```python
from build123d import *

# Parameters (mm, degrees)
BOSS_EXTRUDE1_DEPTH = 4
SKETCH3_R           = 3.1
CUT_EXTRUDE1_DEPTH  = 1
SKETCH4_R           = 2.4
CUT_EXTRUDE2_DEPTH  = 22.365860619
CUT_EXTRUDE4_START  = -1
SKETCH7_R           = 3.1
CUT_EXTRUDE4_DEPTH  = 1
LPATTERN3_COUNT     = 3
LPATTERN3_PITCH     = 8
CUT_EXTRUDE5_DEPTH  = 22.365860619
LPATTERN4_COUNT     = 2
LPATTERN4_PITCH     = 8


with BuildPart() as part:
    # Sketch2 → Boss-Extrude1 (new, symmetric)
    with BuildSketch(Plane(origin=(0, 0, 0), x_dir=(1, 0, 0), z_dir=(0, 1, 0))):
        with BuildLine():
            Line((0, 3.5), (16, 3.5))
            ThreePointArc((16, 3.5), (19.5, 0), (16, -3.5))
            Line((16, -3.5), (0, -3.5))
            ThreePointArc((0, -3.5), (-3.5, 0), (0, 3.5))
        make_face()
    extrude(amount=BOSS_EXTRUDE1_DEPTH, both=True)

    # Sketch3 → Cut-Extrude1 (cut)
    with BuildSketch(Plane(origin=(0, 4, 0), x_dir=(1, 0, 0), z_dir=(0, 1, 0))):
        with Locations(Location((0, 0, 0), (0, 0, 270))):
            Circle(SKETCH3_R)
    cut_extrude1 = extrude(amount=-CUT_EXTRUDE1_DEPTH, mode=Mode.SUBTRACT)

    # Sketch4 → Cut-Extrude2 (cut, through all)
    with BuildSketch(Plane(origin=(0, 4, 0), x_dir=(1, 0, 0), z_dir=(0, 1, 0))):
        with Locations(Location((0, 0, 0), (0, 0, 270))):
            Circle(SKETCH4_R)
    cut_extrude2 = extrude(amount=-CUT_EXTRUDE2_DEPTH, mode=Mode.SUBTRACT)

    # Sketch7 → Cut-Extrude4 (cut)
    with BuildSketch(Plane(origin=(0, -4, 0), x_dir=(-1, 0, 0), z_dir=(0, -1, 0)).offset(CUT_EXTRUDE4_START)):
        with Locations(Location((0, 0, 0), (0, 0, 270))):
            Circle(SKETCH7_R)
    cut_extrude4 = extrude(amount=CUT_EXTRUDE4_DEPTH, mode=Mode.SUBTRACT)

    # LPattern3: Cut-Extrude1, Cut-Extrude2, Cut-Extrude4 ×3
    with Locations(*[(i * LPATTERN3_PITCH, 0, 0) for i in range(1, LPATTERN3_COUNT)]):
        add(cut_extrude1, mode=Mode.SUBTRACT)
        add(cut_extrude2, mode=Mode.SUBTRACT)
        add(cut_extrude4, mode=Mode.SUBTRACT)

    # Sketch8 → Cut-Extrude5 (cut, through all)
    with BuildSketch(Plane(origin=(0, 4, 0), x_dir=(1, 0, 0), z_dir=(0, 1, 0))):
        with BuildLine():
            Line((2.814249456, 3.1), (5.185750544, 3.1))
            ThreePointArc((5.185750544, 3.1), (5.553697029, 2.856892908), (5.474391514, 2.423076923))
            ThreePointArc((5.474391514, 2.423076923), (4.5, 0), (5.474391514, -2.423076923))
            ThreePointArc((5.474391514, -2.423076923), (5.553697029, -2.856892908), (5.185750544, -3.1))
            Line((5.185750544, -3.1), (2.814249456, -3.1))
            ThreePointArc((2.814249456, -3.1), (2.446302971, -2.856892908), (2.525608486, -2.423076923))
            ThreePointArc((2.525608486, -2.423076923), (3.5, 0), (2.525608486, 2.423076923))
            ThreePointArc((2.525608486, 2.423076923), (2.446302971, 2.856892908), (2.814249456, 3.1))
        make_face()
    cut_extrude5 = extrude(amount=-CUT_EXTRUDE5_DEPTH, mode=Mode.SUBTRACT)

    # LPattern4: Cut-Extrude5 ×2
    with Locations(*[(i * LPATTERN4_PITCH, 0, 0) for i in range(1, LPATTERN4_COUNT)]):
        add(cut_extrude5, mode=Mode.SUBTRACT)


solid = part.part
```
Verification items for the finished model (mm, model axes). A direction names the side the tool comes from. Coordinates: 2 decimals unless noted, no trailing zeros. Loops run counter-clockwise (first coordinate to the right, second up) from the corner with the lowest first, then second, coordinate; pieces in that order, holes last. Notation, with made-up numbers: (76, -9) - (102, -9) arc R29 ccw to (102, 24) - close; hole circle Ø2 at (-8, 82.25). An arc over 180 degrees is marked (long way). Put each result on its own line as item: value.
Item 1: Gauge pin test, flat ends, axial feed: pin 1 Ø1.5 at (y, z) = (-3, 1) entering from +X; pin 2 Ø3 at (x, z) = (8.5, -1) entering from -Y. Record the tip position at first contact, or that the pin passes through.
Conclusion:
pin 1: stops at x = 19.49
pin 2: stops at y = -3
Item 2: Section check B-B (y = -0.5). Enter the section's corners in (x, z), then the cut area to 3 significant figures.
Conclusion:
outline: (0, -3.5) - (16, -3.5) arc R3.5 ccw to (16, 3.5) - (0, 3.5) arc R3.5 ccw to start; hole circle Ø4.8 at (0, 0); hole (2.53, -2.42) arc R0.4 ccw to (2.81, -3.1) - (5.19, -3.1) arc R0.4 ccw to (5.47, -2.42) arc R3.5 cw to (5.47, 2.42) arc R0.4 ccw to (5.19, 3.1) - (2.81, 3.1) arc R0.4 ccw to (2.53, 2.42) arc R3.5 cw to start; hole circle Ø4.8 at (8, 0); hole (10.53, -2.42) arc R0.4 ccw to (10.81, -3.1) - (13.19, -3.1) arc R0.4 ccw to (13.47, -2.42) arc R3.5 cw to (13.47, 2.42) arc R0.4 ccw to (13.19, 3.1) - (10.81, 3.1) arc R0.4 ccw to (10.53, 2.42) arc R3.5 cw to start; hole circle Ø4.8 at (16, 0)
area: 72.4 mm2
Item 3: Scan lines: line 1 along X through (y, z) = (-1, 0); line 2 along X through (y, z) = (-3.45, 0); line 3 along Z through (x, y) = (0, -3.5). Record each from-to range of solid material in increasing order.
Conclusion:
line 1: x = -3.5 to -2.4, 2.4 to 3.5, 4.5 to 5.6, 10.4 to 11.5, 12.5 to 13.6, 18.4 to 19.5
line 2: x = -3.5 to -3.1, 3.1 to 3.5, 4.5 to 4.9, 11.1 to 11.5, 12.5 to 12.9, 19.1 to 19.5
line 3: z = -3.5 to -3.1, 3.1 to 3.5
Item 4: Set-up check for faces 1 (the face through (6, 3, 2)), 2 (the face through (4.5, 0.1, 0)), 3 (the face through (18, -3, 2)), 4 (the face through (10, -4, -3)), 5 (the face through (10, 4, -3)): record each of +Z, -Z, +X, -X, +Y, -Y from which the full face is reachable in a straight line by a thin tool's end or side.
Conclusion:
face 1: +Y
face 2: +Y, -Y
face 3: -Y
face 4: +Z, -Z, +X, -X, -Y
face 5: +Z, -Z, +X, -X, +Y
Item 5: Section check C-C (z = 0). Give the number of separate pieces and of enclosed holes in the cut face, then the cut area to 3 significant figures.
Conclusion:
separate pieces: 6
enclosed holes: 0
area: 44.4 mm2
Item 6: Section check D-D (x = -1.75). Enter the section's corners in (y, z), then the cut area to 3 significant figures.
Conclusion:
outline: (-4, -3.03) - (4, -3.03) - (4, -2.56) - (3, -2.56) - (3, -1.64) - (-3, -1.64) - (-3, -2.56) - (-4, -2.56) - close; (-4, 2.56) - (-3, 2.56) - (-3, 1.64) - (3, 1.64) - (3, 2.56) - (4, 2.56) - (4, 3.03) - (-4, 3.03) - close
area: 18.6 mm2
Item 7: Section check A-A (x = 8). Enter the section's corners in (y, z).
Conclusion:
outline: (-4, -3.5) - (4, -3.5) - (4, -3.1) - (3, -3.1) - (3, -2.4) - (-3, -2.4) - (-3, -3.1) - (-4, -3.1) - close; (-4, 3.1) - (-3, 3.1) - (-3, 2.4) - (3, 2.4) - (3, 3.1) - (4, 3.1) - (4, 3.5) - (-4, 3.5) - close
Item 8: Draft check along X on faces 6 (the face through (19.026, -3.493, -0.672)), 7 (the face through (19.5, 0.1, -0.1)), 8 (the face through (8, 0, 3.5)). Enter one of: pulls with the +X half, pulls with the -X half, needs draft (parallel to the pull), parting line crosses it, or undercut.
Conclusion:
face 6: undercut
face 7: pulls with the +X half
face 8: needs draft
